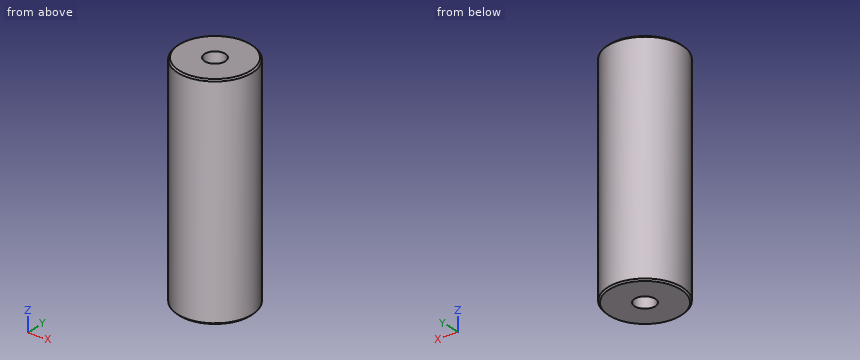
from build123d import *

# Parameters (mm, degrees)
SKETCH1_R           = 12.7
BOSS_EXTRUDE1_DEPTH = 37.75
CHAMFER1_SIZE       = 0.5


with BuildPart() as part:
    # Sketch1 → Boss-Extrude1 (new, symmetric)
    with BuildSketch(Plane.XY):
        Circle(SKETCH1_R)
    extrude(amount=BOSS_EXTRUDE1_DEPTH, both=True)

    # Sketch2 → M8x1.0 Tapped Hole1 (revolve, cut)
    with BuildSketch(Plane(origin=(0, 0, 37.75), x_dir=(0, -1, 0), z_dir=(1, 0, 0))):
        Polygon((0, 0), (0, 14.103012167), (3.5, 12), (3.5, 0), align=None)
    m8x1_0_tapped_hole1 = revolve(axis=Axis((0, 0, 44.1), (0, 0, -1)), mode=Mode.SUBTRACT)

    # Mirror1: M8x1.0 Tapped Hole1 across plane
    add(m8x1_0_tapped_hole1.mirror(Plane.XY), mode=Mode.SUBTRACT)

    # Chamfer1
    chamfer1_edges = [part.edges().sort_by_distance(p)[0] for p in [
        (-12.7, 0, -37.75),
        (-12.7, 0, 37.75),
    ]]
    chamfer(chamfer1_edges, length=CHAMFER1_SIZE)


solid = part.part
Here's how the part is built. I have some questions about the finished solid (model axes, mm). Give positions to 0.01 mm unless a question says otherwise; leave off trailing zeros. Order: outer loops, then holes, each group sorted by start corner. A loop starts at its lowest first (then second) coordinate and runs counter-clockwise, first axis right, second up. Notation, with made-up numbers: (30, 43) -> (53, 43) arc R7 cw to (53, 52) -> close; hole circle Ø11 at (-33.75, 3.25). An arc over 180 degrees is marked (long way). Use a Markdown table: item, result. Add a question column.
Item 1: Imagine slicing it at B-B on z = -2.5. Please give me the cut outline in (x, y).
Item 2: Imagine slicing it at A-A on z = 27. Please give me the cut outline in (x, y), plus the area to 3 significant figures.
Item 3: I need wall thicknesses on line 1 (Y direction, x = 0, z = 32.5); line 2 (Y direction, x = 0, z = -25.5); line 3 (Z direction, x = -2.5, y = -0.5). Which ranges of each line are inside material? Lowest first, please.
Item 4: Will these pins go through, and if not, where does the flat tip stop? pin 1 (6 mm diameter, centred on y = 5, z = 15.5, fed in from -X); pin 2 (11 mm diameter, centred on x = 0, y = 0, fed in from +Z); pin 3 (10 mm diameter, centred on y = -9, z = 17, fed in from -X); pin 4 (1 mm diameter, centred on y = 8.5, z = -13, fed in from -X).
Data:
| question | item | result |
|---|---|---|
| 1 | outline | circle Ø25.4 at (0, 0) |
| 2 | outline | circle Ø25.4 at (0, 0); hole circle Ø7 at (0, 0) |
| 2 | area | 468 mm² |
| 3 | line 1 | y = -12.7 to -3.5, 3.5 to 12.7 |
| 3 | line 2 | y = -12.7 to -3.08, 3.08 to 12.7 |
| 3 | line 3 | z = -25.18 to 25.18 |
| 4 | pin 1 | stops at x = -12.54 |
| 4 | pin 2 | stops at z = 37.75 |
| 4 | pin 3 | stops at x = -12.05 |
| 4 | pin 4 | stops at x = -9.86 |
